Geometry: final body of the model. Coordinates: model frame, mm. Face numbers are marked on the shaded views. A direction names the side the tool comes from. Give positions to 0.01 mm unless a question says otherwise; leave off trailing zeros. Order: outer loops, then holes, each group sorted by start corner. A loop starts at its lowest first (then second) coordinate and runs counter-clockwise, first axis right, second up. Notation, with made-up numbers: (43, 28) -> (89, 28) arc R19 cw to (89, 54) -> close; hole circle Ø2 at (-14.5, 40). An arc over 180 degrees is marked (long way). One line per question, with ' | ' between items. Start each with the question number.
(1) Section B-B (x = 31). Return loops of the section in (y, z), then the cut area to 3 significant figures.
(2) Set-up query: the marked faces 1, 2, 3, 4 and 5. Return all of +Z, -Z, +X, -X, +Y, -Y with unobstructed straight access to the full face (end or side cutting, diameter ignored); none if empty.
(3) Section D-D (y = 37). Return loops of the section in (x, z), then the cut area to 4 significant figures.
(4) First-contact query: pin 1 Ø4 at (y, z) = (10, 16) entering from -X; pin 2 Ø2 at (x, z) = (19, 3.5) entering from +Y; pin 3 Ø3 at (y, z) = (39.5, 15.5) entering from -X; pin 4 Ø6.5 at (y, z) = (26, 3.5) entering from +X. Flat tips, straight axial feed; report the tip coordinate or a pass-through.
(5) Section A-A (z = 12.5). Return loops of the section in (x, y), then the cut area to 3 significant figures.
(6) Ray query, L1, parallel to Y at x = 40.2, z = -15.5; L2, parallel to X at y = 3.25, z = 0; L3, parallel to X at y = 8, z = -19. Return the intervals inside material, ascending.
(7) Mould query, pull axis Y, two halves, no side actions, for the marked faces 6, 7, 8 and 9. Classes: +Y half, -Y half, draft (parallel to the pull), parting line (faces both ways), or undercut.
(8) Section C-C (y = 28.5). State how many separate pieces and enclosed holes the cut face has, then the cut area to 3 significant figures.
Autodesk Inventor part; units mm, degrees
ref_plane "YZ Plane" through (0, 0, 0) normal (1, 0, 0) x (0, 1, 0)
ref_plane "XZ Plane" through (0, 0, 0) normal (0, 1, 0) x (-1, 0, 0)
ref_plane "XY Plane" through (0, 0, 0) normal (0, 0, 1) x (1, 0, 0)
sketch "Sketch3" plane through (0, 0, 0) normal (0, 0, 1) x (1, 0, 0)
  line L0 (0, 0) -> (0, 35)
  line L1 (0, 35) -> (3, 35)
  line L2 (3, 35) -> (3, 4)
  line L3 (3, 4) -> (38, 4)
  line L4 (38, 4) -> (38, 0)
  line L5 (38, 0) -> (0, 0)
  line L6 (0, 25) -> (3, 25) construction
  dimension "d0" = 10
  dimension "d1" = 25
  dimension "d2" = 35
  dimension "d3" = 4
  dimension "d4" = 3
extrude "Extrusion1" add sketch "Sketch3" along normal mid plane 22
sketch "Sketch4" plane through (3, 4, -11) normal (1, 0, 0) x (0, 0, -1)
  line L0 (0, 31) -> (-22, 31) construction
  line L1 (-11, 31) -> (-11, 20) construction
  circle A0 centre (-11, 20) radius 8.05
  point P0 (-11, -4)
  dimension "d7" = 11
  dimension "d8" = 16.1
extrude "Extrusion2" cut sketch "Sketch4" against normal through all
fillet "Fillet3" radius 8 1 edges at (3, 4, 0)
sketch "Sketch5" plane through (3, 4, -11) normal (0, 1, 0) x (1, 0, 0)
  line L0 (35, 0) -> (35, -22) construction
  line L1 (35, -11) -> (0, -11) construction
  line L2 (0, 0) -> (0, -22) construction
  circle A0 centre (7, -11) radius 2.6
  circle A1 centre (28, -11) radius 2.6
  point P0 (-3, -11)
  dimension "d11" = 7
  dimension "d12" = 7
  dimension "d13" = 5.2
extrude "Extrusion3" cut sketch "Sketch5" along normal mid plane 24.75
sketch "Sketch6" plane through (0, 0, 0) normal (0, 0, 1) x (1, 0, 0)
  line L0 (3, 15.95) -> (0, 15.95) construction
  line L1 (0, 15.95) -> (0, 17.95)
  line L2 (0, 17.95) -> (1, 17.95)
  line L3 (1, 17.95) -> (1, 15.95)
  line L4 (0, 15.95) -> (0, 32.05) construction
  line L5 (1, 15.95) -> (0, 15.95)
  line L6 (3, 32.05) -> (3, 15.95) construction
  line L7 (3, 15.95) -> (6, 15.95)
  line L8 (6, 15.95) -> (6, 14.95)
  line L9 (6, 14.95) -> (3, 13.45)
  line L10 (3, 13.45) -> (3, 15.95)
  line L11 (0, 24) -> (3, 24) construction
  point P0 (0, 0)
  dimension "d16" = 1
  dimension "d17" = 2
  dimension "d18" = 5
  dimension "d19" = 2.5
  dimension "d20" = 1
revolve "Revolution1" add sketch "Sketch6" angle 360 about axis through (0, 24, 0) along (1, 0, 0)
fillet "Fillet1" radius 11 2 edges at (1.5, 35, 11) (1.5, 35, -11)
sketch "Sketch7" plane through (38, 0, 11) normal (1, 0, 0) x (0, 0, -1)
  circle A0 centre (11, 24) radius 6.05 construction
  line L0 (-10.25, 2.75) -> (32.25, 2.75) construction
  line L1 (32.25, 2.75) -> (32.25, 45.25)
  line L2 (32.25, 45.25) -> (-10.25, 45.25)
  line L3 (-10.25, 45.25) -> (-10.25, 2.75)
  line L4 (-10.25, 2.75) -> (32.25, 45.25) construction
  line L5 (32.25, 2.75) -> (-10.25, 45.25) construction
  line L6 (-10.25, 2.75) -> (-10.25, 0)
  line L7 (-10.25, 0) -> (32.25, 0)
  line L8 (32.25, 0) -> (32.25, 2.75)
  line L9 (22, 0) -> (0, 0)
  circle A1 centre (11, 24) radius 11
  line L10 (26.5, 8.5) -> (-4.5, 8.5) construction
  line L11 (-4.5, 8.5) -> (-4.5, 39.5) construction
  line L12 (-4.5, 39.5) -> (26.5, 39.5) construction
  line L13 (26.5, 39.5) -> (26.5, 8.5) construction
  line L14 (26.5, 8.5) -> (-4.5, 39.5) construction
  line L15 (-4.5, 8.5) -> (26.5, 39.5) construction
  circle A2 centre (-4.5, 39.5) radius 1.75
  circle A3 centre (-4.5, 8.5) radius 1.75
  circle A4 centre (26.5, 8.5) radius 1.75
  circle A5 centre (26.5, 39.5) radius 1.75
  point P0 (11, 0)
  point P1 (11, 0)
  dimension "d23" = 42.5
  dimension "d24" = 22
  dimension "d25" = 31
  dimension "d26" = 3.5
extrude "Extrusion4" add sketch "Sketch7" along normal blind 5
sketch "Sketch8" plane through (38, 0, 11) normal (-1, 0, 0) x (0, 0, 1)
  line L0 (10.25, 0) -> (0, 0)
  line L1 (0, 0) -> (0, 4)
  line L2 (0, 4) -> (10.25, 4)
  line L3 (10.25, 4) -> (10.25, 0)
  line L4 (-22, 4) -> (-22, 0)
  line L5 (-32.25, 0) -> (-32.25, 45.25)
  line L6 (-22, 4) -> (-32.25, 4)
  line L7 (-32.25, 4) -> (-32.25, 0)
  line L8 (-32.25, 0) -> (-22, 0)
  line L9 (-22, 0) -> (-22, 4)
  point P0 (-11, 0)
extrude "Extrusion5" add sketch "Sketch8" along normal up to surface (38 mm away)
sketch "Sketch9" plane through (38, 4, -21.25) normal (0, 0, -1) x (-1, 0, 0)
  line L0 (0, 9) -> (0, 31)
  line L1 (0, 20.8923) -> (25.405, 0)
  line L2 (0, 0) -> (38, 0)
  line L3 (38, 0) -> (0, 31.25)
  line L4 (0, 0) -> (0, 41.25)
  point P0 (38, -4)
  point P1 (0, 28)
  dimension "d31" = 8
  dimension "d40" = 10
extrude "Extrusion6" add sketch "Sketch9" against normal blind 3 contours L0 L4 L3 L2 L1
fillet "Fillet2" radius 4 2 edges at (38, 30.0711, -18.25) (6.2975, 4, -18.25)
mirror "Mirror1" about plane through (0, 0, 0) normal (0, 0, 1) of "Extrusion6", "Fillet2"
sketch "Sketch10" plane through (0, 4, -11) normal (0, 1, 0) x (1, 0, 0)
  circle A0 centre (10, -11) radius 2.6
  circle A1 centre (10, -11) radius 4.5
  point P0 (0, -11)
  dimension "d37" = 9
extrude "Extrusion7" cut sketch "Sketch10" along normal blind 7 contours A0 | A1
fillet "Fillet4" radius 6 2 edges at (40.5, 45.25, 21.25) (40.5, 45.25, -21.25)
properties part number "Winder_driver"
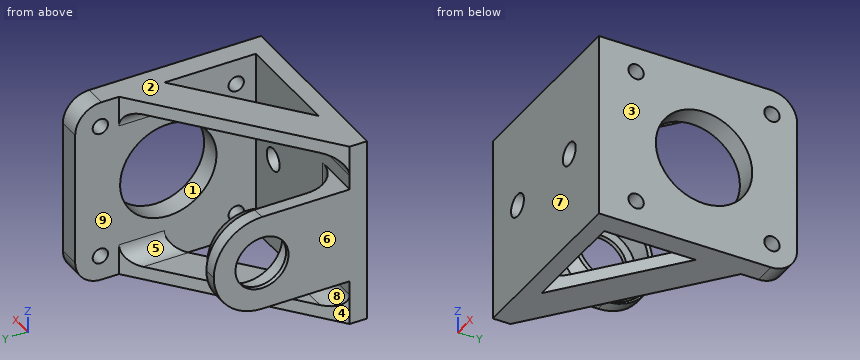
Response:
1) outline: (0, -21.25) -> (4, -21.25) -> (4, -2.6) -> (0, -2.6) -> close; (0, 2.6) -> (4, 2.6) -> (4, 21.25) -> (0, 21.25) -> close; (19.14, -21.25) -> (29.49, -21.25) -> (29.49, -18.25) -> (19.14, -18.25) -> close; (19.14, 18.25) -> (29.49, 18.25) -> (29.49, 21.25) -> (19.14, 21.25) -> close | area: 211 mm^2
2) face 1: +X | face 2: +Z, +X, -X, +Y, -Y | face 3: +Z, -Z, +X, +Y, -Y | face 4: -Z, -X, +Y | face 5: -X, +Y
3) outline: (38, -21.25) -> (43, -21.25) -> (43, 21.25) -> (38, 21.25) -> close | area: 212.5 mm^2
4) pin 1: stops at x = 38 | pin 2: stops at y = 4 | pin 3: passes through | pin 4: stops at x = 1
5) outline: (0, 0) -> (43, 0) -> (43, 45.25) -> (38, 45.25) -> (38, 4) -> (0, 4) -> close | area: 378 mm^2
6) L1: y = 0 to 6.75, 10.25 to 37.75, 41.25 to 45.24 | L2: x = 0 to 7.4, 12.6 to 28.4, 33.6 to 43 | L3: x = 4.86 to 17.46, 38 to 43
7) face 6: draft | face 7: -Y half | face 8: +Y half | face 9: undercut
8) separate pieces: 4 | enclosed holes: 0 | area: 206 mm^2
